```python
from build123d import *

# Parameters (mm, degrees)
F1_DEPTH = 50
F2_R     = 5
F3_R     = 5


with BuildPart() as f1:
    # F0 (on Right) → F1 (new body, symmetric)
    with BuildSketch(Plane.YZ):
        Polygon((300, -10), (320, 10), (-320, 10), (-320, -10), align=None)
        Polygon((-320, -10), (-320, 10), (-390.7106781187, -60.7106781187), (-390.7106781187, -80.7106781187), align=None)
    extrude(amount=F1_DEPTH, both=True)

    # F2
    f2_edges = [f1.edges().sort_by_distance(p)[0] for p in [
        (50, 310, 0),
        (50, 0, 10),
        (50, -355.355339, -25.355339),
        (50, -390.710678, -70.710678),
        (50, -355.355339, -45.355339),
        (50, -10, -10),
        (-50, 310, 0),
        (-50, 0, 10),
        (-50, -355.355339, -25.355339),
        (-50, -390.710678, -70.710678),
        (-50, -355.355339, -45.355339),
        (-50, -10, -10),
    ]]
    fillet(f2_edges, radius=F2_R)

    # F3
    f3_edges = [f1.edges().sort_by_distance(p)[0] for p in [
        (0, -320, 10),
        (0, -390.710678, -60.710678),
    ]]
    fillet(f3_edges, radius=F3_R)


solid = f1.part
```
Input: part model. Units: mm. Frame: model coordinates. A direction names the side the tool comes from. Round coordinates to 2 decimals unless told otherwise and drop trailing zeros. Write each loop counter-clockwise with the first axis right and the second up, starting at its lowest first coordinate (ties: lowest second). Pieces come first, ordered by that corner, then holes. Notation, with made-up numbers: (-20, 61.25) - (-6, 61.25) arc R16 ccw to (-6, 75.25) - close; hole circle Ø7 at (-13, 72). An arc over 180 degrees is marked (long way). Write item = value, one per line.
(1) Contact query for a flat-ended pin moving along its axis: pin 1 Ø3 at (x, y) = (-22, 64) entering from -Z. Output: stop coordinate, or through.
Geometry check:
pin_1 = -10
(2) Section query A-A on x = -32. Output: boundary loops of the cut face in (y, z), then the cut area to 3 significant figures.
Geometry check:
outline = (-390.71, -80.71) - (-320, -10) - (300, -10) - (320, 10) - (-317.93, 10) arc R5 ccw to (-321.46, 8.54) - (-389.25, -59.25) arc R5 ccw to (-390.71, -62.78) - close
area = 14,000 mm^2
(3) Section query B-B on y = 136.5. Output: boundary loops of the cut face in (x, z).
Geometry check:
outline = (-50, -5) arc R5 ccw to (-45, -10) - (45, -10) arc R5 ccw to (50, -5) - (50, 5) arc R5 ccw to (45, 10) - (-45, 10) arc R5 ccw to (-50, 5) - close
(4) Material intervals for probe 1 along Z at (x, y) = (28, -301); probe 2 along X at (y, z) = (-284.5, -9); probe 3 along Y at (x, z) = (-36, -4), sorted ascending.
Geometry check:
probe_1 = -10 to 10
probe_2 = -48 to 48
probe_3 = -334 to 306
(5) Access query for faces 1 (the flat face through (1, -14, -10)), 2 (the cylindrical face through (48.5, -355.13, -43.11)). Directions: +Z, -Z, +X, -X, +Y, -Y. A direction counts if a zero-diameter tool reaches every point of the face in a straight line with its end or side. Return the directions, or none.
Geometry check:
face_1 = -Z, +X, -X, +Y
face_2 = -Z, +X, +Y
